Build history of the part. All positions in model axes, mm. A direction names the side the tool comes from. Round coordinates to 2 decimals unless told otherwise and drop trailing zeros. Loops run counter-clockwise (first coordinate to the right, second up) from the corner with the lowest first, then second, coordinate; pieces in that order, holes last. Notation, with made-up numbers: (82.5, 76) - (141.5, 76) arc R30 cw to (141.5, 98) - close; hole circle Ø6 at (-4, 58). An arc over 180 degrees is marked (long way). Put each result on its own line as item: value. Start each with the question number.
from build123d import *

# Parameters (mm, degrees)
SKETCH1_W           = 20.32
SKETCH1_H           = 38.1
BOSS_EXTRUDE1_DEPTH = 1.5748
FILLET2_R           = 1.27
SKETCH2_W           = 12.192
SKETCH2_H           = 1.772385225
BOSS_EXTRUDE2_DEPTH = 2.54
SKETCH5_W           = 3.750461367
SKETCH5_H           = 13.97
SKETCH5_W_2         = 3.81
BOSS_EXTRUDE3_DEPTH = 7.62
DRAFT2_ANGLE        = 3
DRAFT3_ANGLE        = 3


with BuildPart() as part:
    # Sketch1 → Boss-Extrude1 (new body)
    with BuildSketch(Plane(origin=(0, 0, 0), x_dir=(1, 0, 0), z_dir=(0, 1, 0))):
        with Locations((10.16, 19.05)):
            Rectangle(SKETCH1_W, SKETCH1_H)
    extrude(amount=BOSS_EXTRUDE1_DEPTH)

    # Fillet2
    fillet2_edges = [part.edges().sort_by_distance(p)[0] for p in [
        (0, 0.7874, -38.1),
        (20.32, 0.7874, -38.1),
        (20.32, 0.7874, 0),
        (0, 0.7874, 0),
    ]]
    fillet(fillet2_edges, radius=FILLET2_R)

    # Sketch2 → Boss-Extrude2 (add)
    with BuildSketch(Plane(origin=(0, 1.5748, 0), x_dir=(1, 0, 0), z_dir=(0, 1, 0))):
        with Locations((10.16, 4.097897191)):
            Rectangle(SKETCH2_W, SKETCH2_H)
    extrude(amount=BOSS_EXTRUDE2_DEPTH)

    # Sketch5 → Boss-Extrude3 (add)
    with BuildSketch(Plane(origin=(0, 1.5748, 0), x_dir=(1, 0, 0), z_dir=(0, 1, 0))):
        with Locations((4.474769317, 29.845)):
            Rectangle(SKETCH5_W, SKETCH5_H)
        with Locations((15.875, 29.845)):
            Rectangle(SKETCH5_W_2, SKETCH5_H)
    extrude(amount=BOSS_EXTRUDE3_DEPTH)

    # Draft2
    draft2_faces = [part.faces().sort_by_distance(p)[0] for p in [
        (2.599538633, 5.3848, -29.845),
        (4.474769317, 5.3848, -36.83),
        (6.35, 5.3848, -29.845),
        (4.474769317, 5.3848, -22.86),
    ]]
    draft(draft2_faces, Plane.ZX.offset(1.5748), DRAFT2_ANGLE)

    # Draft3
    draft3_faces = [part.faces().sort_by_distance(p)[0] for p in [
        (15.875, 5.3848, -22.86),
        (13.97, 5.3848, -29.845),
        (15.875, 5.3848, -36.83),
        (17.78, 5.3848, -29.845),
    ]]
    draft(draft3_faces, Plane.ZX.offset(1.5748), DRAFT3_ANGLE)


solid = part.part
Item 1: Slice it at B-B (x = 13.5). Give the cut face in (y, z), plus the area to 3 significant figures.
Item 2: Drop flat-ended pins along their axis: pin 1 Ø1 at (x, y) = (5.5, 8.5) entering from +Z; pin 2 Ø1.3 at (x, y) = (11, 2.5) entering from -Z; pin 3 Ø0.5 at (x, z) = (12, -4.5) entering from +Y; pin 4 Ø3 at (x, y) = (11.5, 8) entering from -Z. Give the stop position or say it passes through.
Item 3: Slice it at D-D (z = -13). Give the cut face in (x, y).
Item 4: Drill centre lines: probe 1 along Z at (x, y) = (11.75, 2); probe 2 along Y at (x, z) = (12.25, -9); probe 3 along Z at (x, y) = (14.5, 3). Where is each one in solid material? Low to high. Write a range as [from, to].
Item 5: Which spindle directions (+Z, -Z, +X, -X, +Y, -Y) get a long thin tool onto all of the face, cutting with end or side? Do faces 4 (the flat face through (4, 9.195, -30)), 5 (the flat face through (6.153, 5.331, -29.747)), 6 (the flat face through (4.449, 5.331, -23.057)), 7 (the flat face through (4.064, 3, -4)). Say none if no direction does.
Item 6: Slice it at A-A (y = 3.75). Give the cut face in (x, z).
Item 7: Two-plate mould, pull along Z, no slides. Class faces 1 (the flat face through (15.848, 5.331, -23.057)), 2 (the flat face through (20.32, 1, -19)), 3 (the cylindrical face through (19.958, 0.798, -37.718)): pulls with the +Z half, pulls with the -Z half, needs draft (parallel to the pull), parting line crosses it, or undercut.
Item 8: Slice it at C-C (z = -26.5). Give the cut face in (x, y).
Computed values:
1. outline: (0, -38.1) - (1.57, -38.1) - (1.57, -4.98) - (4.11, -4.98) - (4.11, -3.21) - (1.57, -3.21) - (1.57, 0) - (0, 0) - close
1. area: 64.5 mm^2
2. pin 1: stops at z = -23.2
2. pin 2: stops at z = -4.98
2. pin 3: stops at y = 4.11
2. pin 4: passes through
3. outline: (0, 0) - (20.32, 0) - (20.32, 1.57) - (0, 1.57) - close
4. probe 1: z = [-4.98, -3.21]
4. probe 2: y = [0, 1.57]
4. probe 3: z = [-36.76, -22.93], [-4.98, -3.21]
5. face 4: +Z, -Z, +X, -X, +Y
5. face 5: -Z, +Y
5. face 6: +X, -X, +Y
5. face 7: +Z, -X, +Y
6. outline: (2.71, -36.72) - (6.24, -36.72) - (6.24, -22.97) - (2.71, -22.97) - close; (4.06, -4.98) - (16.26, -4.98) - (16.26, -3.21) - (4.06, -3.21) - close; (14.08, -36.72) - (17.67, -36.72) - (17.67, -22.97) - (14.08, -22.97) - close
7. face 1: undercut
7. face 2: needs draft
7. face 3: pulls with the -Z half
8. outline: (0, 0) - (20.32, 0) - (20.32, 1.57) - (17.78, 1.57) - (17.38, 9.19) - (14.37, 9.19) - (13.97, 1.57) - (6.35, 1.57) - (5.95, 9.19) - (3, 9.19) - (2.6, 1.57) - (0, 1.57) - close
